Build history of the part. All positions in model axes, mm. A direction names the side the tool comes from. Give positions to 0.01 mm unless a question says otherwise; leave off trailing zeros. Loops run counter-clockwise (first coordinate to the right, second up) from the corner with the lowest first, then second, coordinate; pieces in that order, holes last. Notation, with made-up numbers: (5.5, 25.25) -> (50.5, 25.25) arc R20 ccw to (50.5, 47.25) -> close; hole circle Ø2 at (46, 66.25). An arc over 180 degrees is marked (long way). Answer as a JSON object with one key per item and string values. Group by question number.
Q1. Tool access for faces 1 (the cylindrical face through (20.79, 242.41, 47.99)), 2 (the flat face through (1, -9, 36.5)), 3 (the flat face through (1, -182, 55.748)): list every direction of +Z, -Z, +X, -X, +Y, -Y with a clear straight run to the whole face (end or side of a thin tool).
Q2. Two-plate mould, pull along Y, no slides. Class faces 4 (the flat face through (1, 9, 35.5)), 5 (the flat face through (0.51, -234.92, 51.6)), 6 (the flat face through (0.504, -235.543, 52.393)): pulls with the +Y half, pulls with the -Y half, needs draft (parallel to the pull), parting line crosses it, or undercut.
Q3. Band-saw the part on A-A, the plane x = 126. Write the cut outline in (y, z).
Q4. Wall check: probe 1 along Y at (x, z) = (-242, 36.2); probe 2 along Z at (x, y) = (24, -141.5). Give the ranges that are in metal, low to high. Write a range as from..to.
Q5. Drop flat-ended pins along their axis: pin 1 (2.5 mm diameter, centred on y = -152.5, z = 55.5, fed in from +X); pin 2 (1.5 mm diameter, centred on x = -172.5, z = 38.5, fed in from -Y); pin 3 (1.1 mm diameter, centred on y = 197.5, z = 56.5, fed in from -X); pin 4 (1.1 mm diameter, centred on y = -68, z = 36, fed in from +X). Give the stop position or say it passes through.
from build123d import *

# Parameters (mm, degrees)
SALIENTE_EXTRUIR1_DEPTH     = 271
CORTAR_EXTRUIR9_DEPTH       = 372.074494889
CORTAR_EXTRUIR9_DEPTH_BACK  = 372.074494889
CROQUIS4_R                  = 2.5
CORTAR_EXTRUIR11_DEPTH      = 372.074494889
CORTAR_EXTRUIR11_DEPTH_BACK = 372.074494889
CROQUIS2_W                  = 600.899293422
CROQUIS2_H                  = 554.061756016


with BuildPart() as part:
    # Croquis1 → Saliente-Extruir1 (new, symmetric)
    with BuildSketch(Plane(origin=(0, 0, 0), x_dir=(0, 0, -1), z_dir=(1, 0, 0))):
        Polygon((-36.5, -110), (-36.5, 110), (-56.747809705, 134.130399958), (-56.747809705, 198), (-56.747809705, 228), (-45.747809705, 247.052558883), (-44.881784301, 246.552558883), (-55.747809705, 227.732050808), (-55.747809705, 198), (-55.747809705, 134.494370193), (-35.5, 110.363970234), (-35.5, -110.363970234), (-55.747809705, -134.494370193), (-55.747809705, -198), (-55.747809705, -227.732050808), (-44.881784301, -246.552558883), (-45.747809705, -247.052558883), (-56.747809705, -228), (-56.747809705, -198), (-56.747809705, -134.130399958), align=None)
    extrude(amount=SALIENTE_EXTRUIR1_DEPTH, both=True)

    # Croquis4 → Cortar-Extruir9 (cut, two sides: drawn at the far end of the back side and taken through both)
    with BuildSketch(Plane.XY.offset(-CORTAR_EXTRUIR9_DEPTH_BACK)):
        with Locations(Location((-242, 0, 0), (0, 0, 180))):
            Circle(CROQUIS4_R)
        with Locations(Location((242, 0, 0), (0, 0, 180))):
            Circle(CROQUIS4_R)
        with BuildLine():
            Line((-5, 201.31662479), (-5, 194.68337521))
            ThreePointArc((-5, 194.68337521), (0, 192), (5, 194.68337521))
            Line((5, 194.68337521), (5, 201.31662479))
            ThreePointArc((5, 201.31662479), (0, 204), (-5, 201.31662479))
        make_face()
        with BuildLine():
            Line((5, -201.31662479), (5, -194.68337521))
            ThreePointArc((5, -194.68337521), (0, -192), (-5, -194.68337521))
            Line((-5, -194.68337521), (-5, -201.31662479))
            ThreePointArc((-5, -201.31662479), (0, -204), (5, -201.31662479))
        make_face()
        with BuildLine():
            Line((-5.933205139, 0.892791565), (-3.129872731, -5.118974183))
            ThreePointArc((-3.129872731, -5.118974183), (2.53570957, -5.437846722), (5.933205139, -0.892791565))
            Line((5.933205139, -0.892791565), (3.129872731, 5.118974183))
            ThreePointArc((3.129872731, 5.118974183), (-2.53570957, 5.437846722), (-5.933205139, 0.892791565))
        make_face()
    extrude(amount=CORTAR_EXTRUIR9_DEPTH + CORTAR_EXTRUIR9_DEPTH_BACK, mode=Mode.SUBTRACT)

    # Croquis2 → Cortar-Extruir11 (cut, two sides: drawn at the far end of the back side and taken through both)
    with BuildSketch(Plane.XY.offset(-CORTAR_EXTRUIR11_DEPTH_BACK)):
        Rectangle(CROQUIS2_W, CROQUIS2_H)
        with BuildLine():
            Line((-31.179491924, 174.57413175), (-34.820508076, 180.880556715))
            ThreePointArc((-34.820508076, 180.880556715), (-36.818516526, 185.704175813), (-37.5, 190.880556715))
            Line((-37.5, 190.880556715), (-37.5, 220.353571071))
            ThreePointArc((-37.5, 220.353571071), (-35.939088915, 228.099537764), (-31.5, 234.636427928))
            ThreePointArc((-31.5, 234.636427928), (0, 247.5), (31.5, 234.636427928))
            ThreePointArc((31.5, 234.636427928), (35.939088915, 228.099537764), (37.5, 220.353571071))
            Line((37.5, 220.353571071), (37.5, 190.880556715))
            ThreePointArc((37.5, 190.880556715), (36.818516526, 185.704175813), (34.820508076, 180.880556715))
            Line((34.820508076, 180.880556715), (31.179491924, 174.57413175))
            ThreePointArc((31.179491924, 174.57413175), (29.181483474, 169.750512652), (28.5, 164.57413175))
            Line((28.5, 164.57413175), (28.5, 130.292099447))
            ThreePointArc((28.5, 130.292099447), (29.181483474, 125.115718545), (31.179491924, 120.292099447))
            Line((31.179491924, 120.292099447), (34.820508076, 113.985674482))
            ThreePointArc((34.820508076, 113.985674482), (36.818516526, 109.162055384), (37.5, 103.985674482))
            Line((37.5, 103.985674482), (37.5, 50.768455322))
            ThreePointArc((37.5, 50.768455322), (39.221022598, 36.579915591), (44.28427417, 23.214285714))
            ThreePointArc((44.28427417, 23.214285714), (51.647000448, 15.386930642), (61.997983838, 12.5))
            Line((61.997983838, 12.5), (223.291713066, 12.5))
            ThreePointArc((223.291713066, 12.5), (264.5, 0), (223.291713066, -12.5))
            Line((223.291713066, -12.5), (61.997983838, -12.5))
            ThreePointArc((61.997983838, -12.5), (51.647000448, -15.386930642), (44.28427417, -23.214285714))
            ThreePointArc((44.28427417, -23.214285714), (39.221022598, -36.579915591), (37.5, -50.768455322))
            Line((37.5, -50.768455322), (37.5, -103.985674482))
            ThreePointArc((37.5, -103.985674482), (36.818516526, -109.162055384), (34.820508076, -113.985674482))
            Line((34.820508076, -113.985674482), (31.179491924, -120.292099447))
            ThreePointArc((31.179491924, -120.292099447), (29.181483474, -125.115718545), (28.5, -130.292099447))
            Line((28.5, -130.292099447), (28.5, -164.57413175))
            ThreePointArc((28.5, -164.57413175), (29.181483474, -169.750512652), (31.179491924, -174.57413175))
            Line((31.179491924, -174.57413175), (34.820508076, -180.880556715))
            ThreePointArc((34.820508076, -180.880556715), (36.818516526, -185.704175813), (37.5, -190.880556715))
            Line((37.5, -190.880556715), (37.5, -220.353571071))
            ThreePointArc((37.5, -220.353571071), (35.939088915, -228.099537764), (31.5, -234.636427928))
            ThreePointArc((31.5, -234.636427928), (0, -247.5), (-31.5, -234.636427928))
            ThreePointArc((-31.5, -234.636427928), (-35.939088915, -228.099537764), (-37.5, -220.353571071))
            Line((-37.5, -220.353571071), (-37.5, -190.880556715))
            ThreePointArc((-37.5, -190.880556715), (-36.818516526, -185.704175813), (-34.820508076, -180.880556715))
            Line((-34.820508076, -180.880556715), (-31.179491924, -174.57413175))
            ThreePointArc((-31.179491924, -174.57413175), (-29.181483474, -169.750512652), (-28.5, -164.57413175))
            Line((-28.5, -164.57413175), (-28.5, -130.292099447))
            ThreePointArc((-28.5, -130.292099447), (-29.181483474, -125.115718545), (-31.179491924, -120.292099447))
            Line((-31.179491924, -120.292099447), (-34.820508076, -113.985674482))
            ThreePointArc((-34.820508076, -113.985674482), (-36.818516526, -109.162055384), (-37.5, -103.985674482))
            Line((-37.5, -103.985674482), (-37.5, -50.768455322))
            ThreePointArc((-37.5, -50.768455322), (-39.221022598, -36.579915591), (-44.28427417, -23.214285714))
            ThreePointArc((-44.28427417, -23.214285714), (-51.647000448, -15.386930642), (-61.997983838, -12.5))
            Line((-61.997983838, -12.5), (-223.291713066, -12.5))
            ThreePointArc((-223.291713066, -12.5), (-264.5, 0), (-223.291713066, 12.5))
            Line((-223.291713066, 12.5), (-61.997983838, 12.5))
            ThreePointArc((-61.997983838, 12.5), (-51.647000448, 15.386930642), (-44.28427417, 23.214285714))
            ThreePointArc((-44.28427417, 23.214285714), (-39.221022598, 36.579915591), (-37.5, 50.768455322))
            Line((-37.5, 50.768455322), (-37.5, 103.985674482))
            ThreePointArc((-37.5, 103.985674482), (-36.818516526, 109.162055384), (-34.820508076, 113.985674482))
            Line((-34.820508076, 113.985674482), (-31.179491924, 120.292099447))
            ThreePointArc((-31.179491924, 120.292099447), (-29.181483474, 125.115718545), (-28.5, 130.292099447))
            Line((-28.5, 130.292099447), (-28.5, 164.57413175))
            ThreePointArc((-28.5, 164.57413175), (-29.181483474, 169.750512652), (-31.179491924, 174.57413175))
        make_face(mode=Mode.SUBTRACT)
    extrude(amount=CORTAR_EXTRUIR11_DEPTH + CORTAR_EXTRUIR11_DEPTH_BACK, mode=Mode.SUBTRACT)


solid = part.part
Worked answers:
{
 "1": {"face 1": "+Z, -Z, +X, +Y", "face 2": "+Z, +X, -X", "face 3": "-Z, +X, -X"},
 "2": {"face 4": "needs draft", "face 5": "undercut", "face 6": "pulls with the -Y half"},
 "3": {"outline": "(-12.5, 35.5) -> (12.5, 35.5) -> (12.5, 36.5) -> (-12.5, 36.5) -> close"},
 "4": {"probe 1": "-22.5..-2.5, 2.5..22.5", "probe 2": "55.75..56.75"},
 "5": {"pin 1": "x = 28.5", "pin 2": "through", "pin 3": "x = -37.5", "pin 4": "x = 37.5"}
}
